Source: CAD feature listing. Evaluate the final solid. Frame: model axes, mm. Round coordinates to 2 decimals unless told otherwise and drop trailing zeros. Order: outer loops, then holes, each group sorted by start corner. A loop starts at its lowest first (then second) coordinate and runs counter-clockwise, first axis right, second up. Notation, with made-up numbers: (26, 26) -> (41, 26) arc R8 cw to (41, 32) -> close; hole circle Ø9 at (12, 89.5). An arc over 180 degrees is marked (long way). Answer as CSV lines item,"result". Start each with the question number.
(1) Contact query for flat-ended pins moving along their axis: P1, Ø19, axis at x = -26.5, y = 15, coming from the +Z side; P2, Ø11, axis at x = 16, z = -18, coming from the -Y side. Output: stop coordinate, or through.
(2) Line query: line 1 along Z through (x, y) = (-29.5, -14); line 2 along Z through (x, y) = (14, -15.5); line 3 along Y through (x, z) = (-18, -80.5). Output: solid intervals per line, ascending. Write a range as from..to.
(3) Section query B-B (z = -787). Output: boundary loops of the cut face in (x, y), plus the area to 3 significant figures.
(4) Section query A-A (x = 11). Output: boundary loops of the cut face in (y, z), plus the area to 3 significant figures.
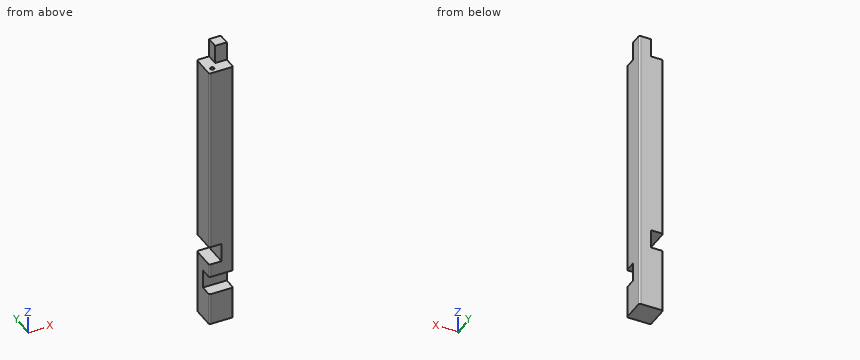
```python
from build123d import *

# Parameters (mm, degrees)
F0_W      = 74
F0_H      = 74
F1_DEPTH  = 900
F2_W      = 74
F2_H      = 58
F4_DEPTH  = 38
F3_W      = 74
F3_H      = 58
F5_DEPTH  = 38
F7_D      = 12
F7_DEPTH  = 40
F7_TIP    = 3.6051637142
F8_W      = 74
F8_H      = 58
F9_DEPTH  = 38
F10_W     = 74
F10_H     = 58
F11_DEPTH = 38
F12_R     = 5


with BuildPart() as f1:
    # F0 (on Top) → F1 (new body)
    with BuildSketch(Plane.XY):
        Rectangle(F0_W, F0_H)
    extrude(amount=-F1_DEPTH)

    # F2 (on face) → F4 (cut)
    with BuildSketch(Plane.XZ.offset(37)):
        with Locations((0, -29)):
            Rectangle(F2_W, F2_H)
    extrude(amount=-F4_DEPTH, mode=Mode.SUBTRACT)

    # F3 (on face) → F5 (cut)
    with BuildSketch(Plane(origin=(-37, 0, 0), x_dir=(0, -1, 0), z_dir=(-1, 0, 0))):
        with Locations((0, -29)):
            Rectangle(F3_W, F3_H)
    extrude(amount=-F5_DEPTH, mode=Mode.SUBTRACT)

    # F7
    with Locations(Plane.XY.offset(-58)):
        with Locations((-18, -18)):
            Hole(F7_D / 2, depth=F7_DEPTH)
            with Locations((0, 0, -(F7_DEPTH + F7_TIP / 2))):  # 118° drill point
                Cone(0, F7_D / 2, F7_TIP, mode=Mode.SUBTRACT)

    # F8 (on face) → F9 (cut)
    with BuildSketch(Plane.XZ.offset(37)):
        with Locations((0, -771)):
            Rectangle(F8_W, F8_H)
    extrude(amount=-F9_DEPTH, mode=Mode.SUBTRACT)

    # F10 (on face) → F11 (cut)
    with BuildSketch(Plane(origin=(-37, 0, 0), x_dir=(0, -1, 0), z_dir=(-1, 0, 0))):
        with Locations((0, -671)):
            Rectangle(F10_W, F10_H)
    extrude(amount=-F11_DEPTH, mode=Mode.SUBTRACT)

    # F12
    f12_edges = [f1.edges().sort_by_distance(p)[0] for p in [
        (-37, -37, -850),
        (-37, -37, -721),
        (-37, -37, -350),
        (-37, 37, -350),
        (-37, 37, -800),
        (37, -37, -850),
        (37, -37, -400),
        (37, 37, -450),
    ]]
    fillet(f12_edges, radius=F12_R)


solid = f1.part
```
Answer block:
1,P1,"z = -58"
1,P2,"y = 1"
2,line 1,"-900..-800, -742..-700, -642..-58"
2,line 2,"-900..-800, -742..-58"
2,line 3,"-37..-24, -12..37"
3,outline,"(-37, 1) -> (37, 1) -> (37, 32) arc R5 ccw to (32, 37) -> (-32, 37) arc R5 ccw to (-37, 32) -> close"
3,area,"2,650 mm2"
4,outline,"(-37, -900) -> (37, -900) -> (37, 0) -> (1, 0) -> (1, -58) -> (-37, -58) -> (-37, -742) -> (1, -742) -> (1, -800) -> (-37, -800) -> close"
4,area,"62,200 mm2"
